Design review of the part built by this model. Coordinates are the model's own, in mm. Give positions to 0.01 mm unless a question says otherwise; leave off trailing zeros. Order: outer loops, then holes, each group sorted by start corner. A loop starts at its lowest first (then second) coordinate and runs counter-clockwise, first axis right, second up.
```python
from build123d import *

# Parameters (mm, degrees)
F0_R     = 7.6537390816
F0_R_2   = 7.7611937188
F0_R_3   = 5.768928847
F0_R_4   = 5.2063685011
F0_R_5   = 9.1585436949
F0_R_6   = 7.6537362484
F0_R_7   = 6.909209466
F0_R_8   = 6
F0_R_9   = 6.061699949
F0_R_10  = 9.524
F0_R_11  = 3.0308412697
F0_R_12  = 10
F1_DEPTH = 8


with BuildPart() as f1:
    # F0 (on Front) → F1 (new body)
    with BuildSketch(Plane.XZ):
        with BuildLine():
            Line((500.7482528687, -20.8750167525), (500.7482528687, 119.1249832475))
            Line((500.7482528687, 119.1249832475), (-63.6194095638, 119.1249832475))
            ThreePointArc((-63.6194095638, 119.1249832475), (-61.3901100274, 117.0030250607), (-60.5691185382, 114.0368059278))
            ThreePointArc((-60.5691185382, 114.0368059278), (-69.3042665181, 109.0888685699), (-69.0566852066, 119.1249832475))
            Line((-69.0566852066, 119.1249832475), (-99.2517471313, 119.1249832475))
            Line((-99.2517471313, 119.1249832475), (-99.2517471313, -20.8750167525))
            Line((-99.2517471313, -20.8750167525), (-34.2517471313, -20.8750167525))
            Line((-34.2517471313, -20.8750167525), (-34.2517471313, 22.1249832475))
            Line((-34.2517471313, 22.1249832475), (21.7482528687, 22.1249832475))
            Line((21.7482528687, 22.1249832475), (21.7482528687, -20.8750167525))
            Line((21.7482528687, -20.8750167525), (500.7482528687, -20.8750167525))
        make_face()
        with Locations((-83.8007479906, -8.2048225315)):
            Circle(F0_R, mode=Mode.SUBTRACT)
        with Locations((-50.4275932908, -7.4259503745)):
            Circle(F0_R_2, mode=Mode.SUBTRACT)
        with Locations((-66.3380473852, 6.9793784816)):
            Circle(F0_R_3, mode=Mode.SUBTRACT)
        with Locations((102.4680286646, -8.5901357234)):
            Circle(F0_R_4, mode=Mode.SUBTRACT)
        with Locations((129.6322196722, 8.8725611567)):
            Circle(F0_R_5, mode=Mode.SUBTRACT)
        with Locations((-48.8753542304, 20.5143652856)):
            Circle(F0_R_6, mode=Mode.SUBTRACT)
        with Locations((-26.7559364438, 37.2009426355)):
            Circle(F0_R_7, mode=Mode.SUBTRACT)
        with Locations((492.7482528687, 4.9516526193)):
            Circle(F0_R_8, mode=Mode.SUBTRACT)
        with Locations((473.7482528687, 14.3054015934)):
            Circle(F0_R_9, mode=Mode.SUBTRACT)
        with Locations((430.7482528687, 49.1249832475)):
            Circle(F0_R_10, mode=Mode.SUBTRACT)
        with Locations((-83.8007479906, 101.2308299541)):
            Circle(F0_R, mode=Mode.SUBTRACT)
        with Locations((248.5129094124, 85.1249832475)):
            Circle(F0_R_11, mode=Mode.SUBTRACT)
        with Locations((263.5129094124, 100.1249832475)):
            Circle(F0_R_12, mode=Mode.SUBTRACT)
        with Locations((278.5129094124, 85.1249832475)):
            Circle(F0_R_11, mode=Mode.SUBTRACT)
        with Locations((301.0329669538, 85.1249832475)):
            Circle(F0_R_11, mode=Mode.SUBTRACT)
        with Locations((331.0329669538, 85.1249832475)):
            Circle(F0_R_11, mode=Mode.SUBTRACT)
        with Locations((316.0329669538, 100.1249832475)):
            Circle(F0_R_12, mode=Mode.SUBTRACT)
        with Locations((248.5129094124, 115.1249832475)):
            Circle(F0_R_11, mode=Mode.SUBTRACT)
        with Locations((278.5129094124, 115.1249832475)):
            Circle(F0_R_11, mode=Mode.SUBTRACT)
        with Locations((301.0329669538, 115.1249832475)):
            Circle(F0_R_11, mode=Mode.SUBTRACT)
        with Locations((331.0329669538, 115.1249832475)):
            Circle(F0_R_11, mode=Mode.SUBTRACT)
        with Locations((492.7482528687, 100.1249832475)):
            Circle(F0_R_8, mode=Mode.SUBTRACT)
        with Locations((473.7482528687, 110.1562082767)):
            Circle(F0_R_9, mode=Mode.SUBTRACT)
        with BuildLine():
            ThreePointArc((-60.5691185382, 114.0368059278), (-61.3901100274, 117.0030250607), (-63.6194095638, 119.1249832475))
            Line((-63.6194095638, 119.1249832475), (-69.0566852066, 119.1249832475))
            ThreePointArc((-69.0566852066, 119.1249832475), (-69.3042665181, 109.0888685699), (-60.5691185382, 114.0368059278))
        make_face()
        with BuildLine():
            Line((-69.0566852066, 119.1249832475), (-63.6194095638, 119.1249832475))
            ThreePointArc((-63.6194095638, 119.1249832475), (-66.3380473852, 119.8057347747), (-69.0566852066, 119.1249832475))
        make_face()
    extrude(amount=F1_DEPTH)


solid = f1.part
```
1. Take a section at B-B (y = -2.5). State how many separate pieces and enclosed holes the cut face has, then the cut area to 3 significant figures.
Recorded:
separate pieces: 1
enclosed holes: 23
area: 78,600 mm2
2. Draft analysis for pull direction X (two halves, no side actions). For faces 1 (the face through (-23, -4, 43)), 2 (the face through (197, -8, 50)), state which applies: pulls with the +X half, pulls with the -X half, needs draft (parallel to the pull), parting line crosses it, or undercut.
Recorded:
face 1: undercut
face 2: needs draft
3. Take a section at A-A (x = 318). State the section outline as (y, z) points, then the cut area to 3 significant figures.
Recorded:
outline: (-8, -20.88) - (0, -20.88) - (0, 90.32) - (-8, 90.32) - close; (-8, 109.93) - (0, 109.93) - (0, 119.12) - (-8, 119.12) - close
area: 963 mm2
4. For line 1 along X through (y, z) = (-4, 15); line 2 along X through (y, z) = (-3.5, 103); line 3 along Z through (x, y) = (361, -6.25), list the stretches that pass through material, from the lowest coordinate up.
Recorded:
line 1: x = -99.25 to -54.18, -43.57 to -34.25, 21.75 to 122.83, 136.44 to 467.73, 479.77 to 500.75
line 2: x = -99.25 to -91.25, -76.35 to 253.94, 273.09 to 306.46, 325.61 to 487.48, 498.01 to 500.75
line 3: z = -20.88 to 119.12
